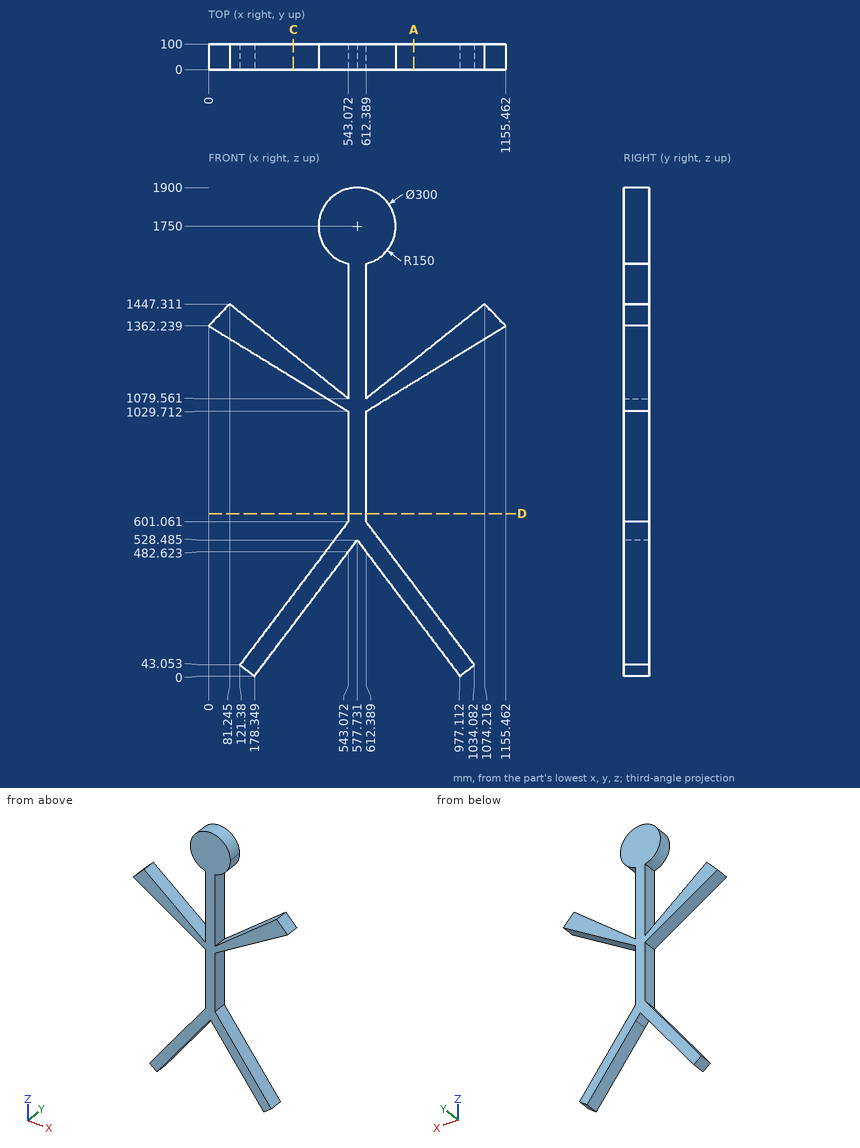
Here's the drawing with two shaded views (mm, measured from the low corner). I have some questions. Round coordinates to 2 decimals unless told otherwise and drop trailing zeros. Loops run counter-clockwise (first coordinate to the right, second up) from the corner with the lowest first, then second, coordinate; pieces in that order, holes last.
Item 1: Suppose I cut it at A-A, the plane x = 798. Write out the boundary of the cut face in (y, z).
Item 2: Will these pins go through, and if not, where does the flat tip stop? pin 1 Ø12 at (x, y) = (565.5, 21.5) entering from -Z; pin 2 Ø4 at (x, y) = (987, 28) entering from +Z (1 decimal); pin 3 Ø2 at (y, z) = (64, 316.5) entering from +X.
Item 3: Suppose I cut it at C-C, the plane x = 329.5. Write out the boundary of the cut face in (y, z).
Item 4: Suppose I cut it at D-D, the plane z = 632. Write out the boundary of the cut face in (x, y), then the cut area to 3 significant figures.
Item 5: Please list where these lines run through material, in increasing order: L1, parallel to Z at x = 713.5, y = 87 (1 decimal); L2, parallel to X at y = 30, z = 708; L3, parallel to X at y = 71, z = 1428 (1 decimal).
Reported:
1. outline: (0, 237.01) - (100, 237.01) - (100, 355.45) - (0, 355.45) - close; (0, 1143.36) - (100, 1143.36) - (100, 1227.36) - (0, 1227.36) - close
2. pin 1: stops at z = 504.36
2. pin 2: stops at z = 1379.5
2. pin 3: stops at x = 828.19
3. outline: (0, 200.01) - (100, 200.01) - (100, 318.45) - (0, 318.45) - close; (0, 1160.48) - (100, 1160.48) - (100, 1249.63) - (0, 1249.63) - close
4. outline: (543.07, 0) - (612.39, 0) - (612.39, 100) - (543.07, 100) - close
4. area: 6,930 mm2
5. L1: z = 348.8 to 467.3, 1091.6 to 1160.1, 1686.2 to 1813.8
5. L2: x = 543.07 to 612.39
5. L3: x = 62.8 to 105.5, 543.1 to 612.4, 1050 to 1092.7
